Work out the finished part from the listing and answer in its coordinate system (mm). Face numbers are marked on the shaded views. A direction names the side the tool comes from. Round coordinates to 2 decimals unless told otherwise and drop trailing zeros. Order: outer loops, then holes, each group sorted by start corner. A loop starts at its lowest first (then second) coordinate and runs counter-clockwise, first axis right, second up.
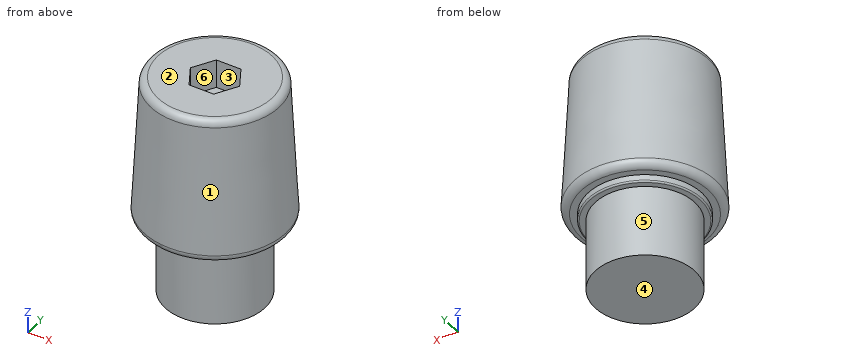
from build123d import *

# Parameters (mm, degrees)
F0_R      = 12.7
F1_DEPTH  = 25.4
F1_TAPER  = 3
F3_DEPTH  = 5.08
F4_R      = 1.27
F5_R      = 1.27
F7_R      = 10.16
F8_DEPTH  = 1.27
F9_R      = 0.254
F10_R     = 8.89
F11_DEPTH = 12.7


with BuildPart() as f1:
    # F0 (on Top) → F1 (new body)
    with BuildSketch(Plane.XY):
        Circle(F0_R)
    extrude(amount=F1_DEPTH, taper=F1_TAPER)

    # F2 (on face) → F3 (cut)
    with BuildSketch(Plane.XY.offset(25.4)):
        Polygon((2.1997045256, 3.81), (-2.1997045256, 3.81), (-4.3994090512, 0), (-2.1997045256, -3.81), (2.1997045256, -3.81), (4.3994090512, 0), align=None)
    extrude(amount=-F3_DEPTH, mode=Mode.SUBTRACT)

    # F4
    f4_edges = [f1.edges().sort_by_distance(p)[0] for p in [
        (-11.368842, 0, 25.4),
    ]]
    fillet(f4_edges, radius=F4_R)

    # F5
    f5_edges = [f1.edges().sort_by_distance(p)[0] for p in [
        (-12.7, 0, 0),
    ]]
    fillet(f5_edges, radius=F5_R)

    # F7 (on face) → F8 (join)
    with BuildSketch(Plane(origin=(0, 0, 0), x_dir=(1, 0, 0), z_dir=(0, 0, -1))):
        Circle(F7_R)
    extrude(amount=F8_DEPTH)

    # F9
    f9_edges = [f1.edges().sort_by_distance(p)[0] for p in [
        (-10.16, 0, -1.27),
    ]]
    fillet(f9_edges, radius=F9_R)

    # F10 (on face) → F11 (join)
    with BuildSketch(Plane(origin=(0, 0, -1.27), x_dir=(1, 0, 0), z_dir=(0, 0, -1))):
        Circle(F10_R)
    extrude(amount=F11_DEPTH)


solid = f1.part
Item 1: For a pull along X with two mould halves and no side action, classify the marked faces 1, 2 and 3 as released by +X, released by -X, zero draft, split by the parting line, or undercut.
Item 2: Given pin 1 (3 mm diameter, centred on x = -7, z = 12.5, fed in from +Y); pin 2 (5 mm diameter, centred on x = -0.5, z = 23, fed in from +Y); pin 3 (2 mm diameter, centred on x = -9.5, y = -6.5, fed in from -Z); pin 4 (6 mm diameter, centred on x = 2, y = 0.5, fed in from +Z), each flat-ended and moving along its own axis, determine where each tip first touches the part or whether it passes through.
Item 3: Find the intervals of material crossed by line 1 along Z through (x, y) = (-9.25, -3); line 2 along Z through (x, y) = (3, -2); line 3 along Y through (x, z) = (6, 5), in increasing order.
Item 4: Find section A-A (x = 0). Write down the section's boundary in (y, z), plus the area to 3 significant figures.
Item 5: Find section C-C (z = 17.5). Write down the section's boundary in (x, y).
Item 6: Find section B-B (z = -7). Write down the section's boundary in (x, y), plus the area to 3 significant figures.
Item 7: A tool of negligible diameter and unlimited length cuts with its end or side. For the marked faces 4, 5 and 6, from which of +Z, -Z, +X, -X, +Y, -Y can it reach the whole face along a straight path? Write none if from no direction.
Model answer:
1. face 1: split by the parting line
1. face 2: zero draft
1. face 3: undercut
2. pin 1: stops at y = 10.72
2. pin 2: stops at y = 11.62
2. pin 3: stops at z = 0
2. pin 4: stops at z = 25.4
3. line 1: z = -1.27 to 25.4
3. line 2: z = -13.97 to 20.32
3. line 3: y = -10.9 to 10.9
4. outline: (-12.63, 1.34) arc R1.27 ccw to (-11.36, 0) - (-10.16, 0) - (-10.16, -1.02) arc R0.25 ccw to (-9.91, -1.27) - (-8.89, -1.27) - (-8.89, -13.97) - (8.89, -13.97) - (8.89, -1.27) - (9.91, -1.27) arc R0.25 ccw to (10.16, -1.02) - (10.16, 0) - (11.36, 0) arc R1.27 ccw to (12.63, 1.34) - (11.43, 24.2) arc R1.27 ccw to (10.16, 25.4) - (3.81, 25.4) - (3.81, 20.32) - (-3.81, 20.32) - (-3.81, 25.4) - (-10.16, 25.4) arc R1.27 ccw to (-11.43, 24.2) - close
4. area: 823 mm2
5. outline: circle Ø23.57 at (0, 0)
6. outline: circle Ø17.78 at (0, 0)
6. area: 248 mm2
7. face 4: -Z, +X, -X, +Y, -Y
7. face 5: -Z
7. face 6: +Z
